Geometry: final body of the model. Coordinates: model frame, mm. Face numbers are marked on the shaded views. A direction names the side the tool comes from. Round coordinates to 2 decimals unless told otherwise and drop trailing zeros. Write each loop counter-clockwise with the first axis right and the second up, starting at its lowest first coordinate (ties: lowest second). Pieces come first, ordered by that corner, then holes. Notation, with made-up numbers: M 53.25,41.25 L 103.25,41.25 A30 cw 103.25,80.25 Z; hole C 61,82.5 d11. An arc over 180 degrees is marked long. Use one line per item in the form item = value. Start each with the question number.
Item 1: Pull-direction query (Y, two-part tool) for the marked faces 1, 2 and 3; classes: pulls with the +Y half, pulls with the -Y half, needs draft (parallel to the pull), parting line crosses it, or undercut.
Item 2: Ray query, probe 1 along X at (y, z) = (3, 3); probe 2 along Y at (x, z) = (-6, 12); probe 3 along X at (y, z) = (2, 6.5). Return the intervals inside material, ascending.
Item 3: Section query A-A (y = 2.75). State how many separate pieces and enclosed holes the cut face has, and give its area (3 significant figures).
Item 4: Section query B-B (z = -2). Return loops of the section in (x, y), and give its area (3 significant figures).
Item 5: Section query C-C (x = 5.5). Return loops of the section in (y, z).
Item 6: Section query D-D (x = -10.5). Return loops of the section in (y, z).
Item 7: Pin query (flat end, axial travel): pin 1 Ø0.5 at (x, y) = (-10, 1) entering from -Z; pin 2 Ø4 at (y, z) = (2, -10.5) entering from +X; pin 3 Ø1.5 at (x, z) = (-2, -9.5) entering from +Y; pin 4 Ø0.5 at (y, z) = (0.5, -7.5) entering from -X. Return the tip coordinate at first contact, or that it passes through.
Item 8: Reachability of the marked faces 4, 5 and 6 from +Z, -Z, +X, -X, +Y, -Y: full face, straight path, thin tool, end or side. Return the list, or none.
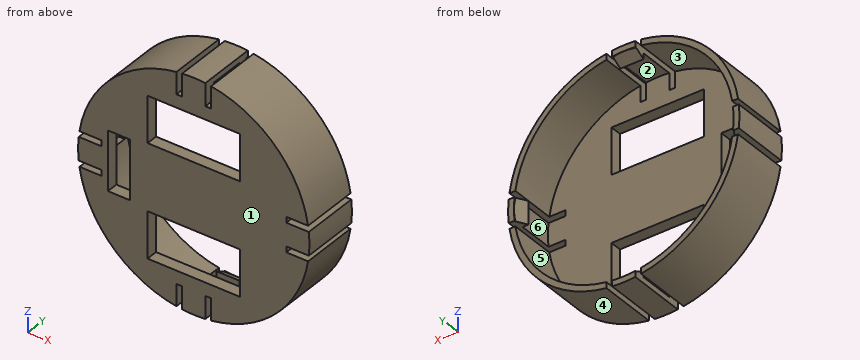
from build123d import *

# Parameters (mm, degrees)
SKETCH1_R           = 15.875
BOSS_EXTRUDE1_DEPTH = 1.5875
BOSS_EXTRUDE2_START = 1.5875
SKETCH1_3_R         = 15.875
SKETCH1_3_R_2       = 15.08125
BOSS_EXTRUDE2_DEPTH = 6.35
CUT_EXTRUDE1_REACH  = 25.812
SKETCH3_W           = 0.79375
SKETCH3_H           = 3.175
BOSS_EXTRUDE3_DEPTH = 1.5875
CIRPATTERN2_COUNT   = 4
SKETCH5_W           = 12.7
SKETCH5_H           = 6.35
SKETCH5_W_2         = 3.048
SKETCH5_H_2         = 8.128
CUT_EXTRUDE2_DEPTH  = 24.3313898


with BuildPart() as part:
    # Sketch1 → Boss-Extrude1 (new body)
    with BuildSketch(Plane(origin=(0, 0, 0), x_dir=(1, 0, 0), z_dir=(0, 1, 0))):
        with Locations(Location((0, 0, 0), (0, 0, 270))):
            Circle(SKETCH1_R)
    extrude(amount=BOSS_EXTRUDE1_DEPTH)

    # Sketch1<3> → Boss-Extrude2 (add)
    with BuildSketch(Plane(origin=(0, 0, 0), x_dir=(1, 0, 0), z_dir=(0, 1, 0)).offset(BOSS_EXTRUDE2_START)):
        with Locations(Location((0, 0, 0), (0, 0, 270))):
            Circle(SKETCH1_3_R)
        with Locations(Location((0, 0, 0), (0, 0, 270))):
            Circle(SKETCH1_3_R_2, mode=Mode.SUBTRACT)
    extrude(amount=BOSS_EXTRUDE2_DEPTH)

    # Cut-Extrude1: up to this face of the body (flat: up to its plane)
    cut_extrude1_end = Plane(part.part.faces().sort_by_distance((0, 0, 0))[0])
    # Sketch3 → Cut-Extrude1 (cut, up to the picked face)
    with BuildSketch(Plane(origin=(0, 7.9375, 0), x_dir=(1, 0, 0), z_dir=(0, 1, 0)), mode=Mode.PRIVATE) as cut_extrude1_sk1:
        with Locations((1.984375, 14.2875)):
            Rectangle(SKETCH3_W, SKETCH3_H)
    cut_extrude1_tool1 = split(extrude(cut_extrude1_sk1.sketch, amount=-CUT_EXTRUDE1_REACH, mode=Mode.PRIVATE), bisect_by=cut_extrude1_end, keep=Keep.BOTH, mode=Mode.PRIVATE)
    # Sketch3 → Cut-Extrude1 (cut, up to the picked face)
    with BuildSketch(Plane(origin=(0, 7.9375, 0), x_dir=(1, 0, 0), z_dir=(0, 1, 0)), mode=Mode.PRIVATE) as cut_extrude1_sk2:
        with Locations((-1.984375, 14.2875)):
            Rectangle(SKETCH3_W, SKETCH3_H)
    cut_extrude1_tool2 = split(extrude(cut_extrude1_sk2.sketch, amount=-CUT_EXTRUDE1_REACH, mode=Mode.PRIVATE), bisect_by=cut_extrude1_end, keep=Keep.BOTH, mode=Mode.PRIVATE)
    cut_extrude1_1 = cut_extrude1_tool1.solids().sort_by(Axis((1.984375, 7.9375, -14.2875), (0, -1, 0)))[0]
    add(cut_extrude1_1, mode=Mode.SUBTRACT)
    cut_extrude1_2 = cut_extrude1_tool2.solids().sort_by(Axis((-1.984375, 7.9375, -14.2875), (0, -1, 0)))[0]
    add(cut_extrude1_2, mode=Mode.SUBTRACT)
    cut_extrude1 = cut_extrude1_1 + cut_extrude1_2  # Cut-Extrude1 as one shape, for the pattern or mirror that repeats it

    # Sketch4 → Boss-Extrude3 (add, symmetric)
    with BuildSketch(Plane.ZY):
        Polygon((-15.795425564, 7.9375), (-15.795425564, 6.4135), (-14.203714629, 6.4135), (-15.08359644, 7.9375), align=None)
    boss_extrude3 = extrude(amount=BOSS_EXTRUDE3_DEPTH, both=True)

    # CirPattern2: Cut-Extrude1, Boss-Extrude3 ×4 about axis
    cirpattern2_axis = Axis((0, 0, 0), (0, 1, 0))
    add([cut_extrude1.rotate(cirpattern2_axis, i * 360 / CIRPATTERN2_COUNT) for i in range(1, CIRPATTERN2_COUNT)], mode=Mode.SUBTRACT)
    add([boss_extrude3.rotate(cirpattern2_axis, i * 360 / CIRPATTERN2_COUNT) for i in range(1, CIRPATTERN2_COUNT)])

    # Sketch5 → Cut-Extrude2 (cut, through all)
    with BuildSketch(Plane(origin=(0, 1.5875, 0), x_dir=(1, 0, 0), z_dir=(0, 1, 0))):
        with Locations((0, 7.7343)):
            Rectangle(SKETCH5_W, SKETCH5_H)
        with Locations((0, -7.7343)):
            Rectangle(SKETCH5_W, SKETCH5_H)
        with Locations((-10.2616, 0)):
            Rectangle(SKETCH5_W_2, SKETCH5_H_2)
    extrude(amount=-CUT_EXTRUDE2_DEPTH, mode=Mode.SUBTRACT)


solid = part.part
Working result:
q1.face_1 = pulls with the -Y half
q1.face_2 = undercut
q1.face_3 = needs draft
q2.probe_1 = -15.59 to -14.78, 14.78 to 15.59
q2.probe_2 = 0 to 1.59
q2.probe_3 = -14.48 to -13.61, 13.61 to 14.48
q3.separate_pieces = 8
q3.enclosed_holes = 0
q3.area = 72.1 mm²
q4.outline = M -12.7,0 L -11.79,0 L -11.79,1.59 L -12.7,1.59 Z; M -8.74,0 L 12.7,0 L 12.7,1.59 L -8.74,1.59 Z
q4.area = 35.5 mm²
q5.outline = M 0,-14.89 L 7.94,-14.89 L 7.94,-14.04 L 1.59,-14.04 L 1.59,-10.91 L 0,-10.91 Z; M 0,-4.56 L 1.59,-4.56 L 1.59,4.56 L 0,4.56 Z; M 0,10.91 L 1.59,10.91 L 1.59,14.04 L 7.94,14.04 L 7.94,14.89 L 0,14.89 Z
q6.outline = M 0,-11.91 L 7.94,-11.91 L 7.94,-10.83 L 1.59,-10.83 L 1.59,-4.06 L 0,-4.06 Z; M 0,4.06 L 1.59,4.06 L 1.59,10.83 L 7.94,10.83 L 7.94,11.91 L 0,11.91 Z
q7.pin_1 = -12.53
q7.pin_2 = 13.41
q7.pin_3 = through
q7.pin_4 = -14.12
q8.face_4 = -Z, +X, +Y, -Y
q8.face_5 = +Y
q8.face_6 = none
